Build history of the part. All positions in model axes, mm. Face numbers are marked on the shaded views. A direction names the side the tool comes from. Round coordinates to 2 decimals unless told otherwise and drop trailing zeros. Order: outer loops, then holes, each group sorted by start corner. A loop starts at its lowest first (then second) coordinate and runs counter-clockwise, first axis right, second up. Notation, with made-up numbers: (40, -36.5) -> (50, -36.5) arc R16 cw to (50, -17.5) -> close; hole circle Ø4 at (4.5, 0.5). An arc over 180 degrees is marked (long way). Use a Markdown table: item, result. Add a question column.
Item 1: Probe L1, parallel to Z at x = 0.8, y = -1.1; L2, parallel to X at y = -0.1, z = 5.25. List the from-to ranges inside material, lowest first.
Item 2: Slice it at A-A, the plane y = 1.35. Give the cut face in (x, z), plus the area to 3 significant figures.
Item 3: 3-axis set-ups, long thin cutter, end or side, ignore diameter. For the marked faces 1 and 2: which of +Z, -Z, +X, -X, +Y, -Y reach the whole face in a straight line?
Item 4: Pin check, flat tips, straight feed: pin 1 (1.5 mm diameter, centred on y = 1, z = 3.5, fed in from -X); pin 2 (0.9 mm diameter, centred on x = -0.5, y = 0, fed in from -Z); pin 3 (1.5 mm diameter, centred on x = 1, z = 1.5, fed in from -Y). Stop position of each tip, or through.
Item 5: Slice it at B-B, the plane x = 0. Give the cut face in (y, z), plus the area to 3 significant figures.
Item 6: Slice it at D-D, the plane z = 8. Give the cut face in (x, y).
Item 7: Two-plate mould, pull along Z, no slides. Class the marked faces 3, 4 and 5: released by +Z, released by -Z, zero draft, split by the parting line, or undercut.
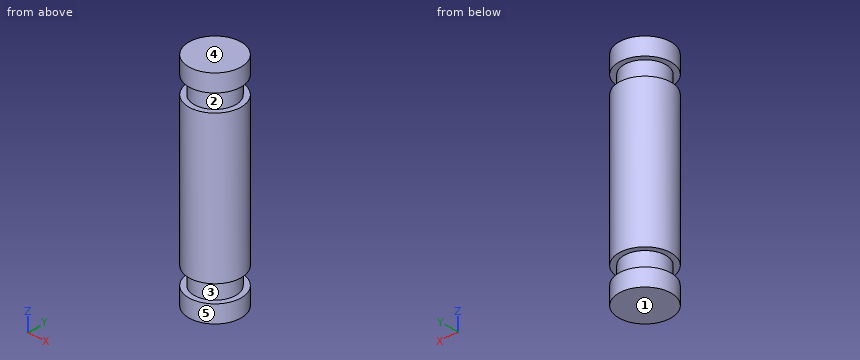
from build123d import *

# Parameters (mm, degrees)
SKETCH1_R           = 1.5
BOSS_EXTRUDE1_DEPTH = 12.5
SKETCH2_W           = 1
SKETCH2_H           = 1.937236023


with BuildPart() as part:
    # Sketch1 → Boss-Extrude1 (new body)
    with BuildSketch(Plane.XY):
        Circle(SKETCH1_R)
    extrude(amount=BOSS_EXTRUDE1_DEPTH)

    # Sketch2 → Cut-Revolve1 (revolve, cut)
    with BuildSketch(Plane(origin=(0, 0, 0), x_dir=(0, 0, -1), z_dir=(1, 0, 0)), mode=Mode.PRIVATE) as cut_revolve1_sk:
        with Locations((-1.5, 2.168618012)):
            Rectangle(SKETCH2_W, SKETCH2_H)
    cut_revolve1 = revolve(cut_revolve1_sk.sketch.rotate(Axis((0, 0, 0), (0, 0, 1)), 90), axis=Axis((0, 0, 0), (0, 0, 1)), mode=Mode.SUBTRACT)

    # Mirror1: Cut-Revolve1 across plane
    add(cut_revolve1.mirror(Plane.XY.offset(6.25)), mode=Mode.SUBTRACT)


solid = part.part
Check sheet entries:
| question | item | result |
|---|---|---|
| 1 | L1 | 0 to 1, 2 to 10.5, 11.5 to 12.5 |
| 1 | L2 | -1.5 to 1.5 |
| 2 | outline | (-0.65, 0) -> (0.65, 0) -> (0.65, 1) -> (-0.65, 1) -> close; (-0.65, 2) -> (0.65, 2) -> (0.65, 10.5) -> (-0.65, 10.5) -> close; (-0.65, 11.5) -> (0.65, 11.5) -> (0.65, 12.5) -> (-0.65, 12.5) -> close |
| 2 | area | 13.7 mm2 |
| 3 | face 1 | -Z, +X, -X, +Y, -Y |
| 3 | face 2 | none |
| 4 | pin 1 | x = -1.48 |
| 4 | pin 2 | z = 0 |
| 4 | pin 3 | y = -1.43 |
| 5 | outline | (-1.5, 0) -> (1.5, 0) -> (1.5, 1) -> (1.2, 1) -> (1.2, 2) -> (1.5, 2) -> (1.5, 10.5) -> (1.2, 10.5) -> (1.2, 11.5) -> (1.5, 11.5) -> (1.5, 12.5) -> (-1.5, 12.5) -> (-1.5, 11.5) -> (-1.2, 11.5) -> (-1.2, 10.5) -> (-1.5, 10.5) -> (-1.5, 2) -> (-1.2, 2) -> (-1.2, 1) -> (-1.5, 1) -> close |
| 5 | area | 36.3 mm2 |
| 6 | outline | circle Ø3 at (0, 0) |
| 7 | face 3 | undercut |
| 7 | face 4 | released by +Z |
| 7 | face 5 | zero draft |
